Input: part model. Units: mm. Frame: model coordinates. A direction names the side the tool comes from. Round coordinates to 2 decimals unless told otherwise and drop trailing zeros. Loops run counter-clockwise (first coordinate to the right, second up) from the corner with the lowest first, then second, coordinate; pieces in that order, holes last. Notation, with made-up numbers: (59.25, 37) - (102.25, 37) arc R21 ccw to (102.25, 50) - close; hole circle Ø6 at (-17, 50). An arc over 180 degrees is marked (long way). Use CSV: the item, a comma, the result in double quotes. Start each with the question number.
1. Pin query (flat end, axial travel): P1, Ø1.5, axis at x = 7, z = 48.5, coming from the -Y side; P2, Ø2, axis at x = -6, y = 21, coming from the -Z side; P3, Ø8, axis at x = 0.5, z = 6.5, coming from the -Y side. Return the tip coordinate at first contact, or that it passes through.
2. Cut plane A-A (x = -16). Return loops of the section in (y, z).
3. Cut plane B-B (z = 4). Return loops of the section in (x, y).
4. Material intervals for probe 1 along Z at (x, y) = (13.5, -16); probe 2 along X at (y, z) = (-0.5, 35); probe 3 along Y at (x, z) = (1, 6.5), sorted ascending. Write a range as from..to.
5. Cut plane C-C (y = 16.5). Return loops of the section in (x, z).
6. Access query for faces 1 (the flat face through (0, -27, 47)), 2 (the cylindrical face through (-3.58, -28.5, 50.45)), 3 (the flat face through (0, 27, 47)), 4 (the cylindrical face through (-13.887, 10.648, 19.72)). Directions: +Z, -Z, +X, -X, +Y, -Y. A direction counts if a zero-diameter tool reaches every point of the face in a straight line with its end or side. Return the directions, or none.
7. Cut plane D-D (y = 24.5). Return loops of the section in (x, z), and give its area (3 significant figures).
Autodesk Inventor part; units mm, degrees
ref_plane "YZ Plane" through (0, 0, 0) normal (1, 0, 0) x (0, 1, 0)
ref_plane "XZ Plane" through (0, 0, 0) normal (0, 1, 0) x (-1, 0, 0)
ref_plane "XY Plane" through (0, 0, 0) normal (0, 0, 1) x (1, 0, 0)
sketch "스케치1" plane through (0, 0, 0) normal (0, 0, 1) x (1, 0, 0)
  circle A0 centre (0, 0) radius 17.5
  dimension "d0" = 35
extrude "돌출1" add sketch "스케치1" along normal blind 40
sketch "스케치2" plane through (0, 0, 40) normal (0, 0, 1) x (1, 0, 0)
  circle A0 centre (0, 1.233) radius 27.5
  point P0 (0, 0)
  dimension "d3" = 55
  dimension "d4" = 1.233
extrude "돌출2" add sketch "스케치2" along normal blind 7
sketch "스케치3" plane through (0, 1.233, 47) normal (0, 0, 1) x (1, 0, 0)
  circle A0 centre (0, -1.233) radius 17.5 construction
  circle A1 centre (0, -1.233) radius 17.5 construction
  circle A2 centre (0, -1.233) radius 17.5 construction
  circle A3 centre (0, -2.466) radius 27.5
  dimension "d7" = 1.233
  dimension "d8" = 55
extrude "돌출3" add sketch "스케치3" along normal blind 7
properties part number "input_shaft"
Established:
1,P1,"stops at y = -28.01"
1,P2,"stops at z = 40"
1,P3,"stops at y = -17.5"
2,outline,"(-23.6, 47) - (-21.13, 47) - (-21.13, 40) - (-7.09, 40) - (-7.09, 0) - (7.09, 0) - (7.09, 40) - (23.6, 40) - (23.6, 47) - (21.13, 47) - (21.13, 54) - (-23.6, 54) - close"
3,outline,"circle Ø35 at (0, 0)"
4,probe 1,"z = 40..54"
4,probe 2,"x = -17.49..17.49"
4,probe 3,"y = -17.47..17.47"
5,outline,"(-22.87, 40) - (-5.83, 40) - (-5.83, 0) - (5.83, 0) - (5.83, 40) - (22.87, 40) - (22.87, 47) - (21.02, 47) - (21.02, 54) - (-21.02, 54) - (-21.02, 47) - (-22.87, 47) - close"
6,face 1,"-Z, -Y"
6,face 2,"+Z"
6,face 3,"+Z, +Y"
6,face 4,"-Z"
7,outline,"(-14.66, 40) - (14.66, 40) - (14.66, 47) - (9.7, 47) - (9.7, 54) - (-9.7, 54) - (-9.7, 47) - (-14.66, 47) - close"
7,area,"341 mm2"
